Can you work these out from the model? Positions are in its coordinate system, mm. A direction names the side the tool comes from. Give positions to 0.01 mm unless a question says otherwise; leave off trailing zeros. Loops run counter-clockwise (first coordinate to the right, second up) from the corner with the lowest first, then second, coordinate; pieces in that order, holes last. Notation, with made-up numbers: M 89.5,-32.5 L 120.5,-32.5 A11 cw 120.5,-23.5 Z; hole C -2.75,17 d5. An arc over 180 degrees is marked long. Put each result on its own line as item: value. Start each with the question number.
1) Imagine slicing it at A-A (y = 37.5). Write out the boundary of the cut face in (x, z).
2) Imagine slicing it at D-D (z = 29.25). Write out the boundary of the cut face in (x, y), then the cut area to 3 significant figures.
3) Imagine slicing it at C-C (y = 11). Write out the boundary of the cut face in (x, z).
4) For P1, Ø4, axis at x = -156.5, y = -38, coming from the +Z side; P2, Ø1, axis at y = -1, z = 19, coming from the +X side; P3, Ø6, axis at x = -57.5, y = 38.5, coming from the +Z side, each with a flat end and sliding along its axis, tell me the tip position at first contact or that it passes through.
5) For faces 1 (the flat face through (-153.863, 31.697, 17.958)), 2 (the flat face through (-62, -31.723, 17.958)), 3 (the flat face through (-154, -37, 21)), 4 (the cylindrical face through (-54.536, -38.936, 19.028)), 5 (the flat face through (-67, -1, 25)), which set-ups out of +Z, -Z, +X, -X, +Y, -Y let a thin tool reach every point of the face, with its end or its side?
6) If we mould it in two halves opening along Y, with no side actions, what happens to faces 6 (the flat face through (-61, -35, 21)), 7 (the flat face through (-153.126, -41.723, 17.958)), 8 (the flat face through (-62.883, 41.723, 17.958)), 9 (the cylindrical face through (-56.34, -35.98, 15.99))? For each: +Y half, -Y half, draft (parallel to the pull), parting line (faces both ways), or undercut.
7) Imagine slicing it at B-B (x = -141). Write out the boundary of the cut face in (y, z).
8) Please list where these lines run through material, in increasing order: line 1 along Y through (x, z) = (-136, 31); line 2 along X through (y, z) = (-13.5, 24); line 3 along Y through (x, z) = (-58, 16). Write a range as from..to.
from build123d import *

# Parameters (mm, degrees)
SKETCH218_W         = 80
SKETCH218_H         = 80
PAD096_DEPTH        = 6
SKETCH219_W         = 82
SKETCH219_H         = 82
SKETCH219_W_2       = 80
SKETCH219_H_2       = 80
PAD097_DEPTH        = 20
SKETCH220_W         = 82
SKETCH220_H         = 82
PAD098_DEPTH        = 1
HOLE010_D           = 4.5
HOLE010_DEPTH       = 24
HOLE010_CBORE_D     = 7.5
HOLE010_CBORE_DEPTH = 4


with BuildPart() as part:
    # Sketch218 → Pad096 (new body)
    with BuildSketch(Plane.XY):
        with BuildLine():
            Line((-41.02059, 41), (40.97941, 41))
            Line((49.139632, 42.42542), (40.97941, 41))
            ThreePointArc((50.860368, 32.57458), (54.92542, 38.360368), (49.139632, 42.42542))
            Line((41, 30.852179), (50.860368, 32.57458))
            Line((41, 30.852179), (41, -30.847821))
            Line((50.86248, -32.574949), (41, -30.847821))
            ThreePointArc((49.13752, -42.425051), (54.925051, -38.36248), (50.86248, -32.574949))
            Line((41, -41), (49.13752, -42.425051))
            Line((41, -41), (-41, -41))
            Line((-49.13752, -42.425051), (-41, -41))
            ThreePointArc((-50.86248, -32.574949), (-54.925051, -38.36248), (-49.13752, -42.425051))
            Line((-50.86248, -32.574949), (-41, -30.847821))
            Line((-41, -30.847821), (-41, 30.843439))
            Line((-41, 30.843439), (-50.864603, 32.575321))
            ThreePointArc((-49.135397, 42.424679), (-54.924679, 38.364603), (-50.864603, 32.575321))
            Line((-41.02059, 41), (-49.135397, 42.424679))
        make_face()
        Rectangle(SKETCH218_W, SKETCH218_H, mode=Mode.SUBTRACT)
    extrude(amount=PAD096_DEPTH)

    # Sketch219 → Pad097 (join)
    with BuildSketch(Plane.XY):
        Rectangle(SKETCH219_W, SKETCH219_H)
        Rectangle(SKETCH219_W_2, SKETCH219_H_2, mode=Mode.SUBTRACT)
    extrude(amount=PAD097_DEPTH)

    # Sketch220 (on Face25 of Pad097) → Pad098 (join)
    with BuildSketch(Plane.XY.offset(20)):
        Rectangle(SKETCH220_W, SKETCH220_H)
    extrude(amount=PAD098_DEPTH)

    # Hole010
    with Locations(Plane.XY.offset(6)):
        with Locations((-50, 37.5), (50, 37.5), (50, -37.5), (-50, -37.5)):
            CounterBoreHole(HOLE010_D / 2, HOLE010_CBORE_D / 2, HOLE010_CBORE_DEPTH, depth=HOLE010_DEPTH)


with BuildPart() as part_1:
    # Body026 placement: moved
    add(part.part.moved(Location((-108, 0, 15))))


solid = part_1.part
Recorded:
1. outline: M -163,15 L -160.25,15 L -160.25,17 L -161.75,17 L -161.75,21 L -163,21 Z; M -155.75,15 L -148,15 L -148,35 L -68,35 L -68,15 L -60.25,15 L -60.25,17 L -61.75,17 L -61.75,21 L -67,21 L -67,36 L -149,36 L -149,21 L -154.25,21 L -154.25,17 L -155.75,17 Z; M -55.75,15 L -53,15 L -53,21 L -54.25,21 L -54.25,17 L -55.75,17 Z
2. outline: M -149,-41 L -67,-41 L -67,41 L -149,41 Z; hole M -148,-40 L -68,-40 L -68,40 L -148,40 Z
2. area: 324 mm²
3. outline: M -149,15 L -148,15 L -148,35 L -68,35 L -68,15 L -67,15 L -67,36 L -149,36 Z
4. P1: z = 17
4. P2: x = -67
4. P3: z = 21
5. face 1: +Z, -Z, -X
5. face 2: +Z, -Z, +X
5. face 3: +Z, -X, +Y, -Y
5. face 4: +Z
5. face 5: +Z, +X
6. face 6: draft
6. face 7: -Y half
6. face 8: +Y half
6. face 9: undercut
7. outline: M -41,15 L -40,15 L -40,35 L 40,35 L 40,15 L 41,15 L 41,36 L -41,36 Z
8. line 1: -41..-40, 40..41
8. line 2: -149..-148, -68..-67
8. line 3: -42.5..-39.75, -35.25..-32.42, 32.42..35.25, 39.75..42.5
